The listing builds one solid part. Answer for the finished solid, in the listing's coordinates (mm). A direction names the side the tool comes from. Coordinates: 2 decimals unless noted, no trailing zeros. Order: outer loops, then holes, each group sorted by start corner. A loop starts at its lowest first (then second) coordinate and runs counter-clockwise, first axis right, second up. Notation, with made-up numbers: (74.25, 40) -> (87.25, 40) arc R19 cw to (87.25, 74) -> close; hole circle Ø3 at (55, 53.5). An arc over 180 degrees is marked (long way). One line per question, with ' | ' between items.
from build123d import *

# Parameters (mm, degrees)
ENL_V_MAT_EXTRU_1_DEPTH = 44.957365708
ENL_V_MAT_EXTRU_2_REACH = 45.957


with BuildPart() as part:
    # Esquisse1 → Révolution1 (revolve)
    with BuildSketch(Plane(origin=(0, 0, 0), x_dir=(-1, 0, 0), z_dir=(0, 1, 0))):
        with BuildLine():
            Line((0, 11.5), (0, 0))
            Line((0, 0), (30, 0))
            Line((30, 0), (27, 3))
            Line((27, 3), (18, 3))
            ThreePointArc((18, 3), (15.25, 5.75), (18, 8.5))
            Line((18, 8.5), (27, 8.5))
            Line((27, 8.5), (30, 11.5))
            Line((30, 11.5), (0, 11.5))
        make_face()
    revolve(axis=Axis((0, 0, 0), (0, 0, 1)))

    # Esquisse2 → Enlèv. mat.-Extru.1 (cut, through all)
    with BuildSketch(Plane(origin=(0, 0, 0), x_dir=(1, 0, 0), z_dir=(0, 0, -1))):
        Polygon((7.6, 4.387862046), (0, 8.775724092), (-7.6, 4.387862046), (-7.6, -4.387862046), (0, -8.775724092), (7.6, -4.387862046), align=None)
    extrude(amount=-ENL_V_MAT_EXTRU_1_DEPTH, mode=Mode.SUBTRACT)

    # Enlèv. mat.-Extru.2: up to this face of the body (flat: up to its plane)
    enl_v_mat_extru_2_end = Plane(part.part.faces().sort_by_distance((26.236324676, 0, 3))[0])
    # Esquisse3 → Enlèv. mat.-Extru.2 (cut, up to the picked face)
    with BuildSketch(Plane.XY.offset(11.5), mode=Mode.PRIVATE) as enl_v_mat_extru_2_sk1:
        Polygon((-14.784455543, -29.107428163), (-17.815544457, -27.357428163), (-5.315544457, -5.706793069), (-2.284455543, -7.456793069), align=None)
    enl_v_mat_extru_2_tool1 = split(extrude(enl_v_mat_extru_2_sk1.sketch, amount=-ENL_V_MAT_EXTRU_2_REACH, mode=Mode.PRIVATE), bisect_by=enl_v_mat_extru_2_end, keep=Keep.BOTH, mode=Mode.PRIVATE)
    add(enl_v_mat_extru_2_tool1.solids().sort_by(Axis((-10.05, -17.407111, 11.5), (0, 0, -1)))[0], mode=Mode.SUBTRACT)


solid = part.part
Item 1: Each of these flat-tipped pins is pushed along its axis until it touches: pin 1 Ø6 at (x, y) = (-18.5, 2.5) entering from -Z; pin 2 Ø1 at (x, z) = (4.5, 3) entering from +Y; pin 3 Ø6 at (y, z) = (7.5, 8.5) entering from +X; pin 4 Ø1 at (y, z) = (5.5, 9.5) entering from -X. Where does it stop, or does it pass through?
Computed values:
pin 1: stops at z = 0 | pin 2: stops at y = 27.14 | pin 3: stops at x = 29.13 | pin 4: stops at x = -27.97
Item 2: Find the intervals of material crossed by L1, parallel to Z at x = -23.5, y = 1.5; L2, parallel to X at y = 4, z = 5.5; L3, parallel to Y at x = -2, z = 1.25, in increasing order.
Computed values:
L1: z = 0 to 3, 8.5 to 11.5 | L2: x = -14.73 to -7.6, 7.6 to 14.73 | L3: y = -28.68 to -7.62, 7.62 to 28.68
Item 3: Section A-A, the plane y = 0 is taken. Give the vertices of the cut face in (x, z), plus the area to 3 significant figures.
Computed values:
outline: (-30, 0) -> (-7.6, 0) -> (-7.6, 11.5) -> (-30, 11.5) -> (-27, 8.5) -> (-18, 8.5) arc R2.75 cw to (-18, 3) -> (-27, 3) -> close; (7.6, 0) -> (30, 0) -> (27, 3) -> (18, 3) arc R2.75 cw to (18, 8.5) -> (27, 8.5) -> (30, 11.5) -> (7.6, 11.5) -> close | area: 341 mm^2
Item 4: Section B-B, the plane z = 4.5 is taken. Give the vertices of the cut face in (x, y), plus the area to 3 significant figures.
Computed values:
outline: (-9.24, -12.51) -> (-5.32, -5.71) -> (-7.6, -4.39) -> (-7.6, 4.39) -> (0, 8.78) -> (7.6, 4.39) -> (7.6, -4.39) -> (0, -8.78) -> (-2.28, -7.46) -> (-6.21, -14.26) arc R15.55 ccw (long way) to start | area: 532 mm^2
Item 5: For faces 4 (the face through (-6, -12, 3)), 5 (the face through (3.853, -6.551, 5.67)), 6 (the face through (-6.552, -14.848, 8.254)), determine the directions among +Z, -Z, +X, -X, +Y, -Y from which every point of the face is accessible in a straight line to the end or side of a thin tool.
Computed values:
face 4: none | face 5: +Z, -Z | face 6: +Z
Item 6: Determine the mould class of faces 1 (the face through (-3.853, 6.551, 5.67)), 2 (the face through (-6, 6, 11.5)), 3 (the face through (14.6, 22.94, 8.69)) for opening direction Y: pulls with the +Y half, pulls with the -Y half, needs draft (parallel to the pull), parting line crosses it, or undercut.
Computed values:
face 1: undercut | face 2: needs draft | face 3: parting line crosses it
Item 7: Section C-C, the plane z = 9.5 is taken. Give the vertices of the cut face in (x, y), plus the area to 3 significant figures.
Computed values:
outline: (-15.49, -23.33) -> (-5.32, -5.71) -> (-7.6, -4.39) -> (-7.6, 4.39) -> (0, 8.78) -> (7.6, 4.39) -> (7.6, -4.39) -> (0, -8.78) -> (-2.28, -7.46) -> (-12.46, -25.08) arc R28 ccw (long way) to start | area: 2,190 mm^2
